Read the model definition and answer for the solid it produces. Units are mm, in the model's axes. Face numbers are marked on the shaded views. A direction names the side the tool comes from. Give positions to 0.01 mm unless a question says otherwise; leave off trailing zeros. Write each loop counter-clockwise with the first axis right and the second up, starting at its lowest first coordinate (ties: lowest second). Pieces come first, ordered by that corner, then holes. Notation, with made-up numbers: (-18.5, -6.5) -> (21.5, -6.5) arc R22 ccw to (21.5, 13.5) -> close; hole circle Ø6 at (45, 42.25). An arc over 180 degrees is marked (long way). Use a Markdown table: item, result.
from build123d import *

# Parameters (mm, degrees)
SKETCH_1_W                = 78
SKETCH_1_H                = 15
EXTRUDE_1_DEPTH           = 3
SKETCH_3_R                = 1.5
CUT_EXTRUDE_1_DEPTH       = 3
SKETCH_4_R                = 6
EXTRUDE_2_DEPTH           = 18
SKETCH_5_R                = 4.5
CUT_EXTRUDE_2_DEPTH       = 21
F_2_0MM_2_D               = 3
F_2_0MM_2_DEPTH           = 4.5
F_2_0MM_2_TIP             = 1.5
F_2_0MM_2_ON_FACE_2_D     = 3
F_2_0MM_2_ON_FACE_2_DEPTH = 4.5
F_2_0MM_2_ON_FACE_2_TIP   = 1.5
SKETCH_10_W               = 6
SKETCH_10_H               = 10
CUT_EXTRUDE_3_DEPTH       = 7
SKETCH_13_W               = 19.835687411
SKETCH_13_H               = 21.610205193
CUT_EXTRUDE_4_DEPTH       = 20
SKETCH_14_W               = 11.523038103
SKETCH_14_H               = 10.49031299
EXTRUDE_3_DEPTH           = 3
SKETCH_18_W               = 78
SKETCH_18_H               = 8
EXTRUDE_4_DEPTH           = 3
SKETCH_19_W               = 36.767904102
SKETCH_19_H               = 2.5
EXTRUDE_5_DEPTH           = 12.5
SKETCH_23_R               = 1.65
CUT_EXTRUDE_6_DEPTH       = 12.5
SKETCH_25_W               = 4.236607592
SKETCH_25_H               = 5.36409187
EXTRUDE_7_DEPTH           = 2.5
SKETCH_26_R               = 1.6
CUT_EXTRUDE_7_DEPTH       = 2.5
SKETCH_27_W               = 21.346012392
SKETCH_27_H               = 6.594354882
EXTRUDE_8_DEPTH           = 2.5
SKETCH_28_W               = 36.767231154
SKETCH_28_H               = 5.91819544
EXTRUDE_9_DEPTH           = 2.5
SKETCH_29_W               = 27.660340415
SKETCH_29_H               = 3.5
CUT_EXTRUDE_9_DEPTH       = 2.5
SKETCH_30_W               = 78
SKETCH_30_H               = 8
CUT_EXTRUDE_10_DEPTH      = 100
SKETCH_31_W               = 60.820132647
SKETCH_31_H               = 3
EXTRUDE_10_DEPTH          = 49
SKETCH_32_W               = 48
SKETCH_32_H               = 3.2
CUT_EXTRUDE_11_DEPTH      = 49
SKETCH_33_W               = 15
SKETCH_33_H               = 49.05968874
CUT_EXTRUDE_12_DEPTH      = 100
SKETCH_34_R               = 4.25
EXTRUDE_11_DEPTH          = 49
SKETCH_35_R               = 6
EXTRUDE_12_DEPTH          = 6
SKETCH_36_W               = 8.5
SKETCH_36_H               = 40
CUT_EXTRUDE_13_DEPTH      = 11
SKETCH_37_R               = 3.25
CUT_EXTRUDE_16_DEPTH      = 100
SKETCH_39_W               = 8.456699936
SKETCH_39_H               = 16
CUT_EXTRUDE_17_DEPTH      = 1.25
F_3_0MM_1_D               = 2.9
F_3_0MM_1_DEPTH           = 4.128752102
F_3_0MM_1_TIP             = 0.871247898
F_3_0MM_2_D               = 2.9
F_3_0MM_2_DEPTH           = 4.128752102
F_3_0MM_2_TIP             = 0.871247898
F_3_0MM_3_D               = 2.9
F_3_0MM_3_DEPTH           = 4.128752102
F_3_0MM_3_TIP             = 0.871247898
SKETCH_46_W               = 13.227107738
SKETCH_46_H               = 4.428434999
EXTRUDE_13_DEPTH          = 46
CUT_EXTRUDE_18_DEPTH      = 55


with BuildPart() as part:
    # Sketch 1 → Extrude 1 (new body)
    with BuildSketch(Plane(origin=(0, 0, 0), x_dir=(1, 0, 0), z_dir=(0, 1, 0))):
        Rectangle(SKETCH_1_W, SKETCH_1_H)
    extrude(amount=EXTRUDE_1_DEPTH)

    # Sketch 3 → Cut-Extrude 1 (cut)
    with BuildSketch(Plane(origin=(0, 3, 0), x_dir=(1, 0, 0), z_dir=(0, 1, 0))):
        with Locations(Location((-34.76, -1.72, 0), (0, 0, 270))):
            Circle(SKETCH_3_R)
        with Locations(Location((-24.35, 4.1, 0), (0, 0, 270))):
            Circle(SKETCH_3_R)
        with Locations(Location((31.56, 4.221692081, 0), (0, 0, 270))):
            Circle(SKETCH_3_R)
        with Locations(Location((7.56, 4.221692081, 0), (0, 0, 270))):
            Circle(SKETCH_3_R)
    extrude(amount=-CUT_EXTRUDE_1_DEPTH, mode=Mode.SUBTRACT)

    # Sketch 4 → Extrude 2 (add)
    with BuildSketch(Plane(origin=(0, 3, 0), x_dir=(1, 0, 0), z_dir=(0, 1, 0))):
        with Locations(Location((-3, -1.234165229, 0), (0, 0, 270))):
            Circle(SKETCH_4_R)
    extrude(amount=EXTRUDE_2_DEPTH)

    # Sketch 5 → Cut-Extrude 2 (cut)
    with BuildSketch(Plane(origin=(0, 21, 0), x_dir=(1, 0, 0), z_dir=(0, 1, 0))):
        with Locations(Location((-3, -1.234165229, 0), (0, 0, 270))):
            Circle(SKETCH_5_R)
    extrude(amount=-CUT_EXTRUDE_2_DEPTH, mode=Mode.SUBTRACT)

    # 2.0mm _2
    with Locations(Plane(origin=(-7.901331048, 17.342107422, 4.694938836), x_dir=(-0.576795601176, 0, -0.816888507977), z_dir=(-0.816888507977, 0, 0.576795601176))):
        with Locations((0, 0)):
            Hole(F_2_0MM_2_D / 2, depth=F_2_0MM_2_DEPTH)
            with Locations((0, 0, -(F_2_0MM_2_DEPTH + F_2_0MM_2_TIP / 2))):  # 90° drill point
                Cone(0, F_2_0MM_2_D / 2, F_2_0MM_2_TIP, mode=Mode.SUBTRACT)

    # 2.0mm _2 on face 2
    with Locations(Plane(origin=(1.071764877, 17.164817099, 5.641061052), x_dir=(0.734483043181, 0, -0.678627039897), z_dir=(0.678627039897, 0, 0.734483043181))):
        with Locations((0, 0)):
            Hole(F_2_0MM_2_ON_FACE_2_D / 2, depth=F_2_0MM_2_ON_FACE_2_DEPTH)
            with Locations((0, 0, -(F_2_0MM_2_ON_FACE_2_DEPTH + F_2_0MM_2_ON_FACE_2_TIP / 2))):  # 90° drill point
                Cone(0, F_2_0MM_2_ON_FACE_2_D / 2, F_2_0MM_2_ON_FACE_2_TIP, mode=Mode.SUBTRACT)

    # Sketch 10 → Cut-Extrude 3 (cut)
    with BuildSketch(Plane(origin=(0, 0, -7.5), x_dir=(-1, 0, 0), z_dir=(0, 0, -1))):
        with Locations((3, 8)):
            Rectangle(SKETCH_10_W, SKETCH_10_H)
    extrude(amount=-CUT_EXTRUDE_3_DEPTH, mode=Mode.SUBTRACT)

    # Sketch 13 → Cut-Extrude 4 (cut)
    with BuildSketch(Plane(origin=(0, 0, -7.5), x_dir=(-1, 0, 0), z_dir=(0, 0, -1))):
        with Locations((3.314421038, 13.805102597)):
            Rectangle(SKETCH_13_W, SKETCH_13_H)
    extrude(amount=-CUT_EXTRUDE_4_DEPTH, mode=Mode.SUBTRACT)

    # Sketch 14 → Extrude 3 (add)
    with BuildSketch(Plane(origin=(0, 3, 0), x_dir=(1, 0, 0), z_dir=(0, 1, 0))):
        with Locations((-2.989467433, -1.263493391)):
            Rectangle(SKETCH_14_W, SKETCH_14_H)
    extrude(amount=-EXTRUDE_3_DEPTH)

    # Sketch 18 → Extrude 4 (add)
    with BuildSketch(Plane.XZ):
        with Locations((0, 11.5)):
            Rectangle(SKETCH_18_W, SKETCH_18_H)
    extrude(amount=-EXTRUDE_4_DEPTH)

    # Sketch 19 → Extrude 5 (add)
    with BuildSketch(Plane.XZ):
        with Locations((0.839237194, 14.25)):
            Rectangle(SKETCH_19_W, SKETCH_19_H)
    extrude(amount=EXTRUDE_5_DEPTH)

    # Sketch 23 → Cut-Extrude 6 (cut)
    with BuildSketch(Plane(origin=(0, 0, 13), x_dir=(-1, 0, 0), z_dir=(0, 0, -1))):
        with Locations((-8.603189245, -6.05592298)):
            Circle(SKETCH_23_R)
        with Locations((2.596810755, -6.05592298)):
            Circle(SKETCH_23_R)
    extrude(amount=-CUT_EXTRUDE_6_DEPTH, mode=Mode.SUBTRACT)

    # Sketch 25 → Extrude 7 (add)
    with BuildSketch(Plane(origin=(0, 0, 13), x_dir=(-1, 0, 0), z_dir=(0, 0, -1))):
        with Locations((2.330668631, -6.426480946)):
            Rectangle(SKETCH_25_W, SKETCH_25_H)
    extrude(amount=-EXTRUDE_7_DEPTH)

    # Sketch 26 → Cut-Extrude 7 (cut)
    with BuildSketch(Plane(origin=(0, 0, 13), x_dir=(-1, 0, 0), z_dir=(0, 0, -1))):
        with Locations((4.196810755, -6.05592298)):
            Circle(SKETCH_26_R)
    extrude(amount=-CUT_EXTRUDE_7_DEPTH, mode=Mode.SUBTRACT)

    # Sketch 27 → Extrude 8 (add)
    with BuildSketch(Plane(origin=(0, 0, 13), x_dir=(-1, 0, 0), z_dir=(0, 0, -1))):
        with Locations((-2.379316694, -6.691741876)):
            Rectangle(SKETCH_27_W, SKETCH_27_H)
    extrude(amount=-EXTRUDE_8_DEPTH)

    # Sketch 28 → Extrude 9 (add)
    with BuildSketch(Plane(origin=(0, 0, 13), x_dir=(-1, 0, 0), z_dir=(0, 0, -1))):
        with Locations((-0.839573668, -15.45909772)):
            Rectangle(SKETCH_28_W, SKETCH_28_H)
    extrude(amount=-EXTRUDE_9_DEPTH)

    # Sketch 29 → Cut-Extrude 9 (cut)
    with BuildSketch(Plane(origin=(0, 0, 13), x_dir=(-1, 0, 0), z_dir=(0, 0, -1))):
        with Locations((-0.633763758, -13.394190827)):
            Rectangle(SKETCH_29_W, SKETCH_29_H)
    extrude(amount=-CUT_EXTRUDE_9_DEPTH, mode=Mode.SUBTRACT)

    # Sketch 30 → Cut-Extrude 10 (cut)
    with BuildSketch(Plane(origin=(0, 3, 0), x_dir=(1, 0, 0), z_dir=(0, 1, 0))):
        with Locations((0, -11.5)):
            Rectangle(SKETCH_30_W, SKETCH_30_H)
    extrude(amount=-CUT_EXTRUDE_10_DEPTH, mode=Mode.SUBTRACT)

    # Sketch 31 → Extrude 10 (add)
    with BuildSketch(Plane.XZ):
        with Locations((0.65611444, 6)):
            Rectangle(SKETCH_31_W, SKETCH_31_H)
    extrude(amount=EXTRUDE_10_DEPTH)

    # Sketch 32 → Cut-Extrude 11 (cut)
    with BuildSketch(Plane(origin=(0, 0, 4.5), x_dir=(-1, 0, 0), z_dir=(0, 0, -1))):
        with Locations((-0.175604554, -15.854114518)):
            Rectangle(SKETCH_32_W, SKETCH_32_H)
        with Locations((-0.205191163, -23.054114518)):
            Rectangle(SKETCH_32_W, SKETCH_32_H)
        with Locations((-0.173277927, -30.254114518)):
            Rectangle(SKETCH_32_W, SKETCH_32_H)
        with Locations((-0.15338956, -37.454114518)):
            Rectangle(SKETCH_32_W, SKETCH_32_H)
        with Locations((-0.189333293, -44.654114518)):
            Rectangle(SKETCH_32_W, SKETCH_32_H)
        with Locations((-0.276259634, -9.654114518)):
            Rectangle(SKETCH_32_W, SKETCH_32_H)
    extrude(amount=-CUT_EXTRUDE_11_DEPTH, mode=Mode.SUBTRACT)

    # Sketch 33 → Cut-Extrude 12 (cut)
    with BuildSketch(Plane(origin=(31.066180764, 0, 0), x_dir=(0, 0, -1), z_dir=(1, 0, 0))):
        with Locations((0, -24.52984437)):
            Rectangle(SKETCH_33_W, SKETCH_33_H)
    extrude(amount=-CUT_EXTRUDE_12_DEPTH, mode=Mode.SUBTRACT)

    # Sketch 34 → Extrude 11 (add)
    with BuildSketch(Plane.XZ):
        with Locations(Location((3, 3.071565001, 0), (0, 0, 90))):
            Circle(SKETCH_34_R)
    extrude(amount=EXTRUDE_11_DEPTH)

    # Sketch 35 → Extrude 12 (add)
    with BuildSketch(Plane.XZ.offset(49)):
        with Locations(Location((3, 3.071565001, 0), (0, 0, 270))):
            Circle(SKETCH_35_R)
    extrude(amount=-EXTRUDE_12_DEPTH)

    # Sketch 36 → Cut-Extrude 13 (cut)
    with BuildSketch(Plane(origin=(0, 0, -7.5), x_dir=(-1, 0, 0), z_dir=(0, 0, -1))):
        with Locations((-3, -20)):
            Rectangle(SKETCH_36_W, SKETCH_36_H)
    extrude(amount=-CUT_EXTRUDE_13_DEPTH, mode=Mode.SUBTRACT)

    # Sketch 37 → Cut-Extrude 16 (cut)
    with BuildSketch(Plane.XZ.offset(49)):
        with Locations(Location((3, 3.071565001, 0), (0, 0, 270))):
            Circle(SKETCH_37_R)
    extrude(amount=-CUT_EXTRUDE_16_DEPTH, mode=Mode.SUBTRACT)

    # Sketch 39 → Cut-Extrude 17 (cut)
    with BuildSketch(Plane(origin=(0, 0, 3.5), x_dir=(-1, 0, 0), z_dir=(0, 0, -1))):
        with Locations((-3, -32)):
            Rectangle(SKETCH_39_W, SKETCH_39_H)
    extrude(amount=-CUT_EXTRUDE_17_DEPTH, mode=Mode.SUBTRACT)

    # 3.0mm _1
    with Locations(Plane(origin=(3.06916604, -45.926554475, -2.928036324), x_dir=(-0.999933554166, 0, -0.011527673319), z_dir=(0.011527673319, 0, -0.999933554166))):
        with Locations((0, 0)):
            Hole(F_3_0MM_1_D / 2, depth=F_3_0MM_1_DEPTH)
            with Locations((0, 0, -(F_3_0MM_1_DEPTH + F_3_0MM_1_TIP / 2))):  # 118° drill point
                Cone(0, F_3_0MM_1_D / 2, F_3_0MM_1_TIP, mode=Mode.SUBTRACT)

    # 3.0mm _2
    with Locations(Plane(origin=(-2.19436254, -45.980907568, 6.074663036), x_dir=(-0.500516339146, 0, -0.865727089936), z_dir=(-0.865727089936, 0, 0.500516339146))):
        with Locations((0, 0)):
            Hole(F_3_0MM_2_D / 2, depth=F_3_0MM_2_DEPTH)
            with Locations((0, 0, -(F_3_0MM_2_DEPTH + F_3_0MM_2_TIP / 2))):  # 118° drill point
                Cone(0, F_3_0MM_2_D / 2, F_3_0MM_2_TIP, mode=Mode.SUBTRACT)

    # 3.0mm _3
    with Locations(Plane(origin=(8.205806468, -46.039954185, 6.054781221), x_dir=(-0.497202703373, 0, 0.86763441135), z_dir=(0.86763441135, 0, 0.497202703373))):
        with Locations((0, 0)):
            Hole(F_3_0MM_3_D / 2, depth=F_3_0MM_3_DEPTH)
            with Locations((0, 0, -(F_3_0MM_3_DEPTH + F_3_0MM_3_TIP / 2))):  # 118° drill point
                Cone(0, F_3_0MM_3_D / 2, F_3_0MM_3_TIP, mode=Mode.SUBTRACT)

    # Sketch 46 → Extrude 13 (add)
    with BuildSketch(Plane(origin=(0, 3, 0), x_dir=(1, 0, 0), z_dir=(0, 1, 0))):
        with Locations((2.976074231, -5.285782501)):
            Rectangle(SKETCH_46_W, SKETCH_46_H)
    extrude(amount=-EXTRUDE_13_DEPTH)

    # Sketch 48 → Cut-Extrude 18 (cut)
    with BuildSketch(Plane.XZ.offset(49)):
        with BuildLine():
            Line((-0.25, 3.071565001), (6.25, 3.071565001))
            ThreePointArc((6.25, 3.071565001), (3, 6.321565001), (-0.25, 3.071565001))
        make_face()
    extrude(amount=-CUT_EXTRUDE_18_DEPTH, mode=Mode.SUBTRACT)


solid = part.part
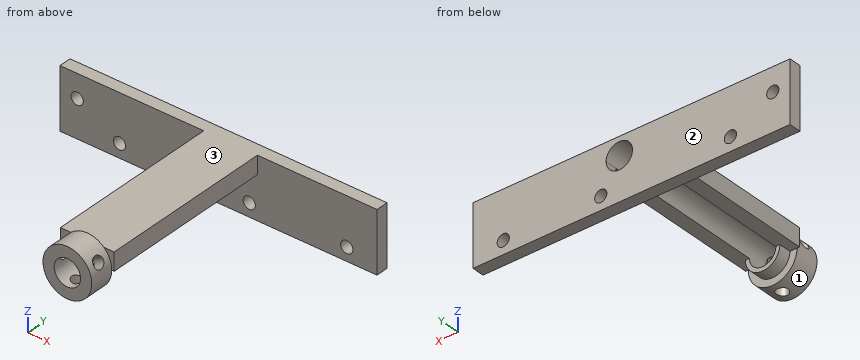
Item 1: A cutting plane is placed at C-C (y = -10.5). Give the vertices of the cut face in (x, z).
Return value:
| item | result |
|---|---|
| outline | (-3.64, 3.07) -> (-0.25, 3.07) arc R3.25 cw to (6.25, 3.07) -> (9.59, 3.07) -> (9.59, 7.5) -> (-3.64, 7.5) -> close |
Item 2: A cutting plane is placed at A-A (x = 31.56). Give the vertices of the cut face in (y, z).
Return value:
| item | result |
|---|---|
| outline | (0, -7.5) -> (3, -7.5) -> (3, -5.72) -> (0, -5.72) -> close; (0, -2.72) -> (3, -2.72) -> (3, 7.5) -> (0, 7.5) -> close |
Item 3: Each of these flat-tipped pins is pushed along its axis until it touches: P1, Ø2, axis at y = -20.5, z = 6, coming from the +X side; P2, Ø14, axis at x = 12, y = -26, coming from the +Z side; P3, Ø3.5, axis at x = 8, y = -18.5, coming from the -Z side. Where does it stop, or does it pass through?
Return value:
| item | result |
|---|---|
| P1 | x = 9.59 |
| P2 | z = 7.5 |
| P3 | z = 3.07 |
Item 4: A cutting plane is placed at B-B (z = -4.5). Give the vertices of the cut face in (x, y).
Return value:
| item | result |
|---|---|
| outline | (-39, 0) -> (-25.8, 0) -> (-25.8, 3) -> (-39, 3) -> close; (-22.9, 0) -> (6.09, 0) -> (6.09, 3) -> (-22.9, 3) -> close; (9.03, 0) -> (30.09, 0) -> (30.09, 3) -> (9.03, 3) -> close; (33.03, 0) -> (39, 0) -> (39, 3) -> (33.03, 3) -> close |
Item 5: A tool of negligible diameter and unlimited length cuts with its end or side. For the marked faces 1, 2 and 3, from which of +Z, -Z, +X, -X, +Y, -Y can it reach the whole face along a straight path? Write none if from no direction.
Return value:
| item | result |
|---|---|
| face 1 | -Y |
| face 2 | +Z, -Z, +X, -X, +Y |
| face 3 | +Z, +X, -X, +Y |
Item 6: Straight lines are drawn through the part: line 1 along X through (y, z) = (1, 1.72); line 2 along X through (y, z) = (-14, 7); line 3 along Z through (x, y) = (31.5, 0.5). For each, find the intervals that lie inside material, in ascending order. Write a range as [from, to].
Return value:
| item | result |
|---|---|
| line 1 | [-39, -36.26], [-33.26, 0.04], [5.96, 39] |
| line 2 | [-3.64, 9.59] |
| line 3 | [-7.5, -5.72], [-2.72, 7.5] |
Item 7: A cutting plane is placed at D-D (z = 1.72). Give the vertices of the cut face in (x, y).
Return value:
| item | result |
|---|---|
| outline | (-39, 0) -> (-36.26, 0) -> (-36.26, 3) -> (-39, 3) -> close; (-33.26, 0) -> (0.04, 0) -> (0.04, 3) -> (-33.26, 3) -> close; (-2.85, -49) -> (0.04, -49) -> (0.04, -40) -> (-1.03, -40) -> (-1.03, -43) -> (-2.85, -43) -> close; (5.96, -49) -> (8.85, -49) -> (8.85, -43) -> (7.03, -43) -> (7.03, -40) -> (5.96, -40) -> close; (5.96, 0) -> (39, 0) -> (39, 3) -> (5.96, 3) -> close |
